```python
from build123d import *

# Parameters (mm, degrees)
SKETCH1_R           = 3
SKETCH1_R_2         = 1.5
BOSS_EXTRUDE1_DEPTH = 2.25
SKETCH2_R           = 3.879501895
BOSS_EXTRUDE2_DEPTH = 2.25
SKETCH3_R           = 3
SKETCH3_R_2         = 2.008527967
BOSS_EXTRUDE3_DEPTH = 1
SKETCH4_R           = 3.8
SKETCH4_R_2         = 3
CUT_EXTRUDE1_DEPTH  = 0.5
SKETCH5_W           = 2
SKETCH5_H           = 45.085962507
BOSS_EXTRUDE4_DEPTH = 2
CUT_EXTRUDE2_START  = -2.25
SKETCH7_R           = 3.879501895
CUT_EXTRUDE2_DEPTH  = 2.25
SKETCH8_R           = 3
SKETCH8_R_2         = 2.5
BOSS_EXTRUDE5_DEPTH = 4
SKETCH9_W           = 2
SKETCH9_H           = 3.166270057
CUT_EXTRUDE3_DEPTH  = 2


with BuildPart() as part:
    # Sketch1 → Boss-Extrude1 (new body)
    with BuildSketch(Plane(origin=(0, 0, 0), x_dir=(1, 0, 0), z_dir=(0, 1, 0))):
        with BuildLine():
            Line((2.2, -54), (6.944444444, -7.195463248))
            ThreePointArc((6.944444444, -7.195463248), (0, 10), (-6.944444444, -7.195463248))
            Line((-6.944444444, -7.195463248), (-2.2, -54))
            ThreePointArc((-2.2, -54), (0, -56.2), (2.2, -54))
        make_face()
        with Locations(Location((0, 0, 0), (0, 0, 270))):
            Circle(SKETCH1_R, mode=Mode.SUBTRACT)
        with Locations(Location((0, -54, 0), (0, 0, 270))):
            Circle(SKETCH1_R_2, mode=Mode.SUBTRACT)
        with Locations(Location((0, -50.5, 0), (0, 0, 270))):
            Circle(SKETCH1_R_2, mode=Mode.SUBTRACT)
    extrude(amount=BOSS_EXTRUDE1_DEPTH)

    # Sketch2 → Boss-Extrude2 (add)
    with BuildSketch(Plane(origin=(0, 2.25, 0), x_dir=(1, 0, 0), z_dir=(0, 1, 0))):
        with Locations(Location((0, 0, 0), (0, 0, 270))):
            Circle(SKETCH2_R)
        with BuildLine():
            Line((1.96, 0), (2.349274052, 0.224747479))
            ThreePointArc((2.349274052, 0.224747479), (2.341390695, 0.295786431), (2.331359713, 0.366554076))
            Line((2.331359713, 0.366554076), (1.898422996, 0.487432179))
            Line((1.898422996, 0.487432179), (2.219574862, 0.801927322))
            ThreePointArc((2.219574862, 0.801927322), (2.194272507, 0.868773944), (2.166957468, 0.934823689))
            Line((2.166957468, 0.934823689), (1.717561093, 0.944237201))
            Line((1.717561093, 0.944237201), (1.950411621, 1.328719123))
            ThreePointArc((1.950411621, 1.328719123), (1.909280107, 1.387173195), (1.866397317, 1.444354892))
            Line((1.866397317, 1.444354892), (1.42877851, 1.341712328))
            Line((1.42877851, 1.341712328), (1.558696845, 1.772022614))
            ThreePointArc((1.558696845, 1.772022614), (1.504320616, 1.818411253), (1.448564558, 1.863131966))
            Line((1.448564558, 1.863131966), (1.050220518, 1.654882734))
            Line((1.050220518, 1.654882734), (1.069043413, 2.103983408))
            ThreePointArc((1.069043413, 2.103983408), (1.004839128, 2.135391844), (0.939713161, 2.164841605))
            Line((0.939713161, 2.164841605), (0.605673309, 1.864070772))
            Line((0.605673309, 1.864070772), (0.512218052, 2.303743186))
            ThreePointArc((0.512218052, 2.303743186), (0.442219902, 2.318197912), (0.371816129, 2.330526285))
            Line((0.371816129, 2.330526285), (0.123069418, 1.956132388))
            Line((0.123069418, 1.956132388), (-0.076791853, 2.358750307))
            ThreePointArc((-0.076791853, 2.358750307), (-0.148185626, 2.355343079), (-0.219443477, 2.349775428))
            Line((-0.219443477, 2.349775428), (-0.367267377, 1.925283011))
            Line((-0.367267377, 1.925283011), (-0.660976643, 2.265548472))
            ThreePointArc((-0.660976643, 2.265548472), (-0.729280107, 2.244493378), (-0.796914643, 2.221379538))
            Line((-0.796914643, 2.221379538), (-0.834527411, 1.773461023))
            Line((-0.834527411, 1.773461023), (-1.20362984, 2.029993894))
            ThreePointArc((-1.20362984, 2.029993894), (-1.264551236, 1.992613904), (-1.324312731, 1.953406202))
            Line((-1.324312731, 1.953406202), (-1.24935102, 1.510205956))
            Line((-1.24935102, 1.510205956), (-1.670654548, 1.666887333))
            ThreePointArc((-1.670654548, 1.666887333), (-1.720365961, 1.61553117), (-1.768499379, 1.562693171))
            Line((-1.768499379, 1.562693171), (-1.585673309, 1.152059094))
            Line((-1.585673309, 1.152059094), (-2.032705886, 1.199044112))
            ThreePointArc((-2.032705886, 1.199044112), (-2.068083765, 1.136938671), (-2.101564707, 1.07379038))
            Line((-2.101564707, 1.07379038), (-1.822361912, 0.721524123))
            Line((-1.822361912, 0.721524123), (-2.267034837, 0.655860539))
            ThreePointArc((-2.267034837, 0.655860539), (-2.28585626, 0.586908134), (-2.302580996, 0.517417391))
            Line((-2.302580996, 0.517417391), (-1.944544815, 0.245653138))
            Line((-1.944544815, 0.245653138), (-2.358917653, 0.071466836))
            ThreePointArc((-2.358917653, 0.071466836), (-2.36, 0), (-2.358917653, -0.071466836))
            Line((-2.358917653, -0.071466836), (-1.944544815, -0.245653138))
            Line((-1.944544815, -0.245653138), (-2.302580996, -0.517417391))
            ThreePointArc((-2.302580996, -0.517417391), (-2.28585626, -0.586908134), (-2.267034837, -0.655860539))
            Line((-2.267034837, -0.655860539), (-1.822361912, -0.721524123))
            Line((-1.822361912, -0.721524123), (-2.101564707, -1.07379038))
            ThreePointArc((-2.101564707, -1.07379038), (-2.068083765, -1.136938671), (-2.032705886, -1.199044112))
            Line((-2.032705886, -1.199044112), (-1.585673309, -1.152059094))
            Line((-1.585673309, -1.152059094), (-1.768499379, -1.562693171))
            ThreePointArc((-1.768499379, -1.562693171), (-1.720365961, -1.61553117), (-1.670654548, -1.666887333))
            Line((-1.670654548, -1.666887333), (-1.24935102, -1.510205956))
            Line((-1.24935102, -1.510205956), (-1.324312731, -1.953406202))
            ThreePointArc((-1.324312731, -1.953406202), (-1.264551236, -1.992613904), (-1.20362984, -2.029993894))
            Line((-1.20362984, -2.029993894), (-0.834527411, -1.773461023))
            Line((-0.834527411, -1.773461023), (-0.796914643, -2.221379538))
            ThreePointArc((-0.796914643, -2.221379538), (-0.729280107, -2.244493378), (-0.660976643, -2.265548472))
            Line((-0.660976643, -2.265548472), (-0.367267377, -1.925283011))
            Line((-0.367267377, -1.925283011), (-0.219443477, -2.349775428))
            ThreePointArc((-0.219443477, -2.349775428), (-0.148185626, -2.355343079), (-0.076791853, -2.358750307))
            Line((-0.076791853, -2.358750307), (0.123069418, -1.956132388))
            Line((0.123069418, -1.956132388), (0.371816129, -2.330526285))
            ThreePointArc((0.371816129, -2.330526285), (0.442219902, -2.318197912), (0.512218052, -2.303743186))
            Line((0.512218052, -2.303743186), (0.605673309, -1.864070772))
            Line((0.605673309, -1.864070772), (0.939713161, -2.164841605))
            ThreePointArc((0.939713161, -2.164841605), (1.004839128, -2.135391844), (1.069043413, -2.103983408))
            Line((1.069043413, -2.103983408), (1.050220518, -1.654882734))
            Line((1.050220518, -1.654882734), (1.448564558, -1.863131966))
            ThreePointArc((1.448564558, -1.863131966), (1.504320616, -1.818411253), (1.558696845, -1.772022614))
            Line((1.558696845, -1.772022614), (1.42877851, -1.341712328))
            Line((1.42877851, -1.341712328), (1.866397317, -1.444354892))
            ThreePointArc((1.866397317, -1.444354892), (1.909280107, -1.387173195), (1.950411621, -1.328719123))
            Line((1.950411621, -1.328719123), (1.717561093, -0.944237201))
            Line((1.717561093, -0.944237201), (2.166957468, -0.934823689))
            ThreePointArc((2.166957468, -0.934823689), (2.194272507, -0.868773944), (2.219574862, -0.801927322))
            Line((2.219574862, -0.801927322), (1.898422996, -0.487432179))
            Line((1.898422996, -0.487432179), (2.331359713, -0.366554076))
            ThreePointArc((2.331359713, -0.366554076), (2.341390695, -0.295786431), (2.349274052, -0.224747479))
            Line((2.349274052, -0.224747479), (1.96, 0))
        make_face(mode=Mode.SUBTRACT)
    extrude(amount=BOSS_EXTRUDE2_DEPTH)

    # Sketch3 → Boss-Extrude3 (add)
    with BuildSketch(Plane.XZ):
        with Locations(Location((0, 0, 0), (0, 0, 270))):
            Circle(SKETCH3_R)
        with Locations(Location((0, 0, 0), (0, 0, 270))):
            Circle(SKETCH3_R_2, mode=Mode.SUBTRACT)
    extrude(amount=-BOSS_EXTRUDE3_DEPTH)

    # Sketch4 → Cut-Extrude1 (cut)
    with BuildSketch(Plane.XZ):
        with Locations(Location((0, 0, 0), (0, 0, 270))):
            Circle(SKETCH4_R)
        with Locations(Location((0, 0, 0), (0, 0, 270))):
            Circle(SKETCH4_R_2, mode=Mode.SUBTRACT)
    extrude(amount=-CUT_EXTRUDE1_DEPTH, mode=Mode.SUBTRACT)

    # Sketch5 → Boss-Extrude4 (add)
    with BuildSketch(Plane(origin=(0, 2.25, 0), x_dir=(1, 0, 0), z_dir=(0, 1, 0))):
        with Locations((0, -26.291385575)):
            Rectangle(SKETCH5_W, SKETCH5_H)
    extrude(amount=BOSS_EXTRUDE4_DEPTH)

    # Sketch7 → Cut-Extrude2 (cut)
    with BuildSketch(Plane(origin=(0, 4.5, 0), x_dir=(1, 0, 0), z_dir=(0, 1, 0)).offset(CUT_EXTRUDE2_START)):
        Circle(SKETCH7_R)
    extrude(amount=CUT_EXTRUDE2_DEPTH, mode=Mode.SUBTRACT)

    # Sketch8 → Boss-Extrude5 (add)
    with BuildSketch(Plane(origin=(0, 1, 0), x_dir=(1, 0, 0), z_dir=(0, 1, 0))):
        with Locations(Location((0, 0, 0), (0, 0, 90))):
            Circle(SKETCH8_R)
        with Locations(Location((0, 0, 0), (0, 0, 270))):
            Circle(SKETCH8_R_2, mode=Mode.SUBTRACT)
    extrude(amount=BOSS_EXTRUDE5_DEPTH)

    # Sketch9 → Cut-Extrude3 (cut)
    with BuildSketch(Plane(origin=(0, 4.25, 0), x_dir=(1, 0, 0), z_dir=(0, 1, 0))):
        with Locations((0, -5.33153935)):
            Rectangle(SKETCH9_W, SKETCH9_H)
    extrude(amount=-CUT_EXTRUDE3_DEPTH, mode=Mode.SUBTRACT)


solid = part.part
```
Part model, mm, in its own coordinate system. A direction names the side the tool comes from. Round coordinates to 2 decimals unless told otherwise and drop trailing zeros. Write each loop counter-clockwise with the first axis right and the second up, starting at its lowest first coordinate (ties: lowest second). Pieces come first, ordered by that corner, then holes.
Item 1: Cut at C-C, the plane x = 0. Count the separate pieces of the cut face and the enclosed holes in it, plus the area to 3 significant figures.
Results:
separate pieces: 4
enclosed holes: 0
area: 211 mm2
Item 2: Drop flat-ended pins along their axis: pin 1 Ø1 at (y, z) = (3, 36) entering from -X; pin 2 Ø4.5 at (x, z) = (0, 0) entering from +Y; pin 3 Ø0.6 at (x, y) = (-0.5, 3.5) entering from -Z. Give the stop position or say it passes through.
Results:
pin 1: stops at x = -1
pin 2: stops at y = 1
pin 3: stops at z = -2.99
Item 3: Cut at D-D, the plane z = 31.5. Give the cut face in (x, y), plus the area to 3 significant figures.
Results:
outline: (-4.48, 0) - (4.48, 0) - (4.48, 2.25) - (1, 2.25) - (1, 4.25) - (-1, 4.25) - (-1, 2.25) - (-4.48, 2.25) - close
area: 24.2 mm2
Item 4: Cut at B-B, the plane z = 0. Give the cut face in (x, y).
Results:
outline: (-10, 0) - (-3.8, 0) - (-3.8, 0.5) - (-3, 0.5) - (-3, 0) - (-2.01, 0) - (-2.01, 1) - (-2.5, 1) - (-2.5, 5) - (-3, 5) - (-3, 2.25) - (-10, 2.25) - close; (2.01, 0) - (3, 0) - (3, 0.5) - (3.8, 0.5) - (3.8, 0) - (10, 0) - (10, 2.25) - (3, 2.25) - (3, 5) - (2.5, 5) - (2.5, 1) - (2.01, 1) - close
Item 5: Probe L1, parallel to X at y = 0.3, z = 0; L2, parallel to X at y = 0.7, z = 0; L3, parallel to Y at x = 0.5, z = 43. List the from-to ranges inside material, lowest first.
Results:
L1: x = -10 to -3.8, -3 to -2.01, 2.01 to 3, 3.8 to 10
L2: x = -10 to -2.01, 2.01 to 10
L3: y = 0 to 4.25
Item 6: Which spindle directions (+Z, -Z, +X, -X, +Y, -Y) get a long thin tool onto all of the face, cutting with end or side? Do faces 1 (the flat face through (0, 3, 48.834)), 2 (the cylindrical face through (-2.44, 2.97, -0.54)), 3 (the flat face through (0, 3, 6.915)). Say none if no direction does.
Results:
face 1: +Z, +X, -X, +Y
face 2: +Y
face 3: +X, -X, +Y
Item 7: Two-plate mould, pull along Z, no slides. Class faces 4 (the cylindrical face through (-1.46, 0.25, -3.51)), 5 (the flat face through (-2, 5, 2)), 6 (the flat face through (4.54, 1.11, 30.93)): +Z half, -Z half, draft (parallel to the pull), parting line (faces both ways), or undercut.
Results:
face 4: undercut
face 5: draft
face 6: +Z half
Item 8: Cut at A-A, the plane y = 2.9. Give the cut face in (x, z).
Results:
outline: circle Ø6 at (0, 0); (-1, 6.91) - (1, 6.91) - (1, 48.83) - (-1, 48.83) - close; hole circle Ø5 at (0, 0)
